```python
from build123d import *

# Parameters (mm, degrees)
SKETCH1_R           = 95
SKETCH1_R_2         = 1.75
BOSS_EXTRUDE1_DEPTH = 2.8
SKETCH2_R           = 4
SKETCH2_R_2         = 2.5
CUT_EXTRUDE1_DEPTH  = 10


with BuildPart() as part:
    # Sketch1 → Boss-Extrude1 (new body)
    with BuildSketch(Plane(origin=(0, 0, 0), x_dir=(1, 0, 0), z_dir=(0, 1, 0))):
        with Locations(Location((0, 0, 0), (0, 0, 270))):
            Circle(SKETCH1_R)
        with Locations(Location((80, 0, 0), (0, 0, 270))):
            Circle(SKETCH1_R_2, mode=Mode.SUBTRACT)
        with Locations(Location((40, -69.282032303, 0), (0, 0, 270))):
            Circle(SKETCH1_R_2, mode=Mode.SUBTRACT)
        with Locations(Location((-40, -69.282032303, 0), (0, 0, 270))):
            Circle(SKETCH1_R_2, mode=Mode.SUBTRACT)
        with Locations(Location((-80, 0, 0), (0, 0, 270))):
            Circle(SKETCH1_R_2, mode=Mode.SUBTRACT)
        with Locations(Location((-40, 69.282032303, 0), (0, 0, 270))):
            Circle(SKETCH1_R_2, mode=Mode.SUBTRACT)
        with Locations(Location((40, 69.282032303, 0), (0, 0, 270))):
            Circle(SKETCH1_R_2, mode=Mode.SUBTRACT)
        with Locations(Location((0, 25, 0), (0, 0, 270))):
            Circle(SKETCH1_R_2, mode=Mode.SUBTRACT)
        with Locations(Location((25, 0, 0), (0, 0, 270))):
            Circle(SKETCH1_R_2, mode=Mode.SUBTRACT)
        with Locations(Location((0, -25, 0), (0, 0, 270))):
            Circle(SKETCH1_R_2, mode=Mode.SUBTRACT)
        with Locations(Location((-25, 0, 0), (0, 0, 270))):
            Circle(SKETCH1_R_2, mode=Mode.SUBTRACT)
    extrude(amount=BOSS_EXTRUDE1_DEPTH)

    # Sketch2 → Cut-Extrude1 (cut)
    with BuildSketch(Plane(origin=(0, 2.8, 0), x_dir=(1, 0, 0), z_dir=(0, 1, 0))):
        with Locations(Location((0, 0, 0), (0, 0, 270))):
            Circle(SKETCH2_R)
        with Locations(Location((11.313708499, 11.313708499, 0), (0, 0, 270))):
            Circle(SKETCH2_R_2)
        with Locations(Location((-11.313708499, -11.313708499, 0), (0, 0, 270))):
            Circle(SKETCH2_R_2)
    extrude(amount=-CUT_EXTRUDE1_DEPTH, mode=Mode.SUBTRACT)


solid = part.part
```
Part model, mm, in its own coordinate system. Coordinates: 2 decimals unless noted, no trailing zeros. Loops run counter-clockwise (first coordinate to the right, second up) from the corner with the lowest first, then second, coordinate; pieces in that order, holes last. Notation, with made-up numbers: (45.5, -37) - (51.5, -37) arc R8 cw to (51.5, -25) - close; hole circle Ø4 at (18, 11). An arc over 180 degrees is marked (long way). Write item = value, one per line. Start each with the question number.
Item 1: Cut at C-C, the plane x = 54. Give the cut face in (y, z), and give its area (3 significant figures).
Item 2: Mould opens along X. For faces 1 (the flat face through (1, 2.8, 20)), 2 (the cylindrical face through (-92.74, 1.38, -20.59)), 3 (the cylindrical face through (-3.905, 1.42, -0.867)) say: released by +X, released by -X, zero draft, split by the parting line, or undercut.
Item 3: Flat gauge pins, fed straight in: pin 1 Ø1 at (y, z) = (2, -13) entering from -X; pin 2 Ø1.5 at (y, z) = (0.5, 29.5) entering from -X. Where does each tip first touch, or does it go through?
Item 4: Wall check: L1, parallel to X at y = 0.85, z = -69; L2, parallel to X at y = 0.7, z = -68; L3, parallel to Z at x = -80, y = 1.3. Give the ranges that are in metal, low to high. Write a range as from..to.
Item 5: Cut at A-A, the plane y = 2.35. State how many separate pieces and enclosed holes the cut face has, and give its area (3 significant figures).
Item 6: Cut at B-B, the plane z = 38.5. Give the cut face in (x, y).
The answers:
q1.outline = (0, -78.16) - (2.8, -78.16) - (2.8, 78.16) - (0, 78.16) - close
q1.area = 438 mm2
q2.face_1 = zero draft
q2.face_2 = split by the parting line
q2.face_3 = undercut
q3.pin_1 = -94.17
q3.pin_2 = -90.55
q4.L1 = -65.3..-41.73, -38.27..38.27, 41.73..65.3
q4.L2 = -66.34..-41.19, -38.81..38.81, 41.19..66.34
q4.L3 = -51.23..-1.75, 1.75..51.23
q5.separate_pieces = 1
q5.enclosed_holes = 13
q5.area = 28,200 mm2
q6.outline = (-86.85, 0) - (86.85, 0) - (86.85, 2.8) - (-86.85, 2.8) - close
